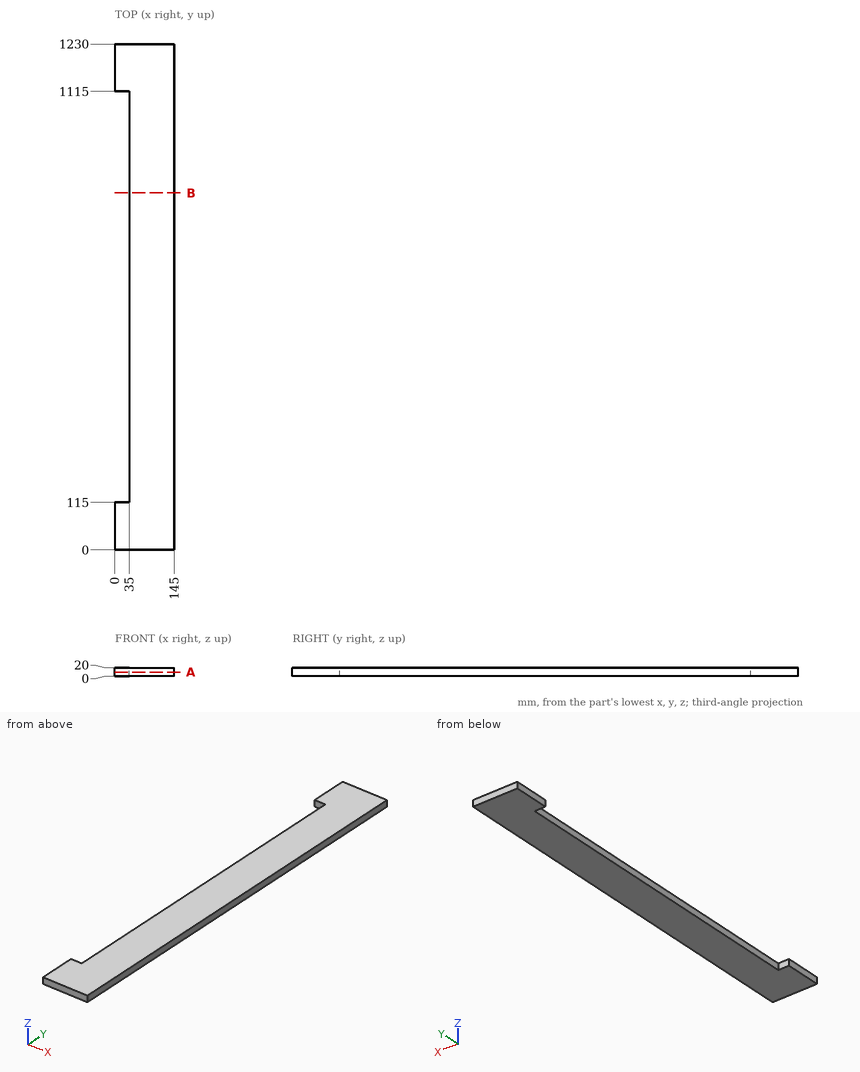
For this review, use the dimensioned drawing (mm, ordinates from the lowest corner) and the shaded views. Round coordinates to 2 decimals unless told otherwise and drop trailing zeros. Write each loop counter-clockwise with the first axis right and the second up, starting at its lowest first coordinate (ties: lowest second). Pieces come first, ordered by that corner, then holes. Notation, with made-up numbers: (37, 24) -> (49, 24) arc R7 cw to (49, 32) -> close; hole circle Ø1 at (2.25, 24.5). An arc over 180 degrees is marked (long way). Use CSV: the item, a comma, the result in double quotes.
Q1. Consider section A-A (z = 9.25). Give the boundary of the cut face in (x, y).
Checks:
outline,"(0, 0) -> (145, 0) -> (145, 1230) -> (0, 1230) -> (0, 1115) -> (35, 1115) -> (35, 115) -> (0, 115) -> close"
Q2. Consider section B-B (y = 868). Give the boundary of the cut face in (x, z), then the cut area to 3 significant figures.
Checks:
outline,"(35, 0) -> (145, 0) -> (145, 20) -> (35, 20) -> close"
area,"2,200 mm²"
Q3. For pin 1 Ø12 at (y, z) = (825, 8.5) entering from -X, flat-tipped, find the tip position at first contact; note if it passes through.
Checks:
pin 1,"x = 35"
Q4. To check wall thickness, follow probe 1 along Y at (x, z) = (19.5, 2.5); probe 2 along X at (y, z) = (470, 6). State the ranges of each line that lie inside material, in increasing order. Write a range as [from, to].
Checks:
probe 1,"[0, 115], [1115, 1230]"
probe 2,"[35, 145]"
